Source: CAD feature listing. Evaluate the final solid. Frame: model axes, mm. A direction names the side the tool comes from. Give positions to 0.01 mm unless a question says otherwise; leave off trailing zeros. Order: outer loops, then holes, each group sorted by start corner. A loop starts at its lowest first (then second) coordinate and runs counter-clockwise, first axis right, second up.
```python
from build123d import *

# Parameters (mm, degrees)
SKETCH1_W           = 203.2
SKETCH1_H           = 152.4
BOSS_EXTRUDE1_DEPTH = 63.5
SKETCH2_W           = 196.85
SKETCH2_H           = 146.05
CUT_EXTRUDE1_DEPTH  = 60.325
SKETCH5_W           = 2.54
SKETCH5_H           = 5.08
CUT_EXTRUDE3_DEPTH  = 47.625
LPATTERN1_COUNT     = 26
LPATTERN1_PITCH     = 7.62
SKETCH6_R           = 8.75
CUT_EXTRUDE4_DEPTH  = 47.625
LPATTERN2_COUNT     = 3
LPATTERN2_PITCH     = 73.66
SKETCH7_R           = 9.525
CUT_EXTRUDE6_DEPTH  = 47.625
SKETCH8_R           = 9.525
CUT_EXTRUDE7_DEPTH  = 47.625


with BuildPart() as part:
    # Sketch1 → Boss-Extrude1 (new body)
    with BuildSketch(Plane(origin=(0, 0, 0), x_dir=(1, 0, 0), z_dir=(0, 1, 0))):
        Rectangle(SKETCH1_W, SKETCH1_H)
    extrude(amount=BOSS_EXTRUDE1_DEPTH)

    # Sketch2 → Cut-Extrude1 (cut)
    with BuildSketch(Plane(origin=(0, 63.5, 0), x_dir=(1, 0, 0), z_dir=(0, 1, 0))):
        Rectangle(SKETCH2_W, SKETCH2_H)
    extrude(amount=-CUT_EXTRUDE1_DEPTH, mode=Mode.SUBTRACT)

    # Sketch5 → Cut-Extrude3 (cut)
    with BuildSketch(Plane.XY.offset(76.2)):
        with Locations((-95.25, 20.32)):
            Rectangle(SKETCH5_W, SKETCH5_H)
    cut_extrude3 = extrude(amount=-CUT_EXTRUDE3_DEPTH, mode=Mode.SUBTRACT)

    # LPattern1: Cut-Extrude3 ×26
    with Locations(*[(i * LPATTERN1_PITCH, 0, 0) for i in range(1, LPATTERN1_COUNT)]):
        add(cut_extrude3, mode=Mode.SUBTRACT)

    # Sketch6 → Cut-Extrude4 (cut)
    with BuildSketch(Plane.XY.offset(76.2)):
        with Locations((-76.2, 44.45)):
            Circle(SKETCH6_R)
    cut_extrude4 = extrude(amount=-CUT_EXTRUDE4_DEPTH, mode=Mode.SUBTRACT)

    # LPattern2: Cut-Extrude4 ×3
    with Locations(*[(i * LPATTERN2_PITCH, 0, 0) for i in range(1, LPATTERN2_COUNT)]):
        add(cut_extrude4, mode=Mode.SUBTRACT)

    # Sketch7 → Cut-Extrude6 (cut)
    with BuildSketch(Plane(origin=(101.6, 0, 0), x_dir=(0, 0, -1), z_dir=(1, 0, 0))):
        with Locations((57.15, 19.05)):
            Circle(SKETCH7_R)
    extrude(amount=-CUT_EXTRUDE6_DEPTH, mode=Mode.SUBTRACT)

    # Sketch8 → Cut-Extrude7 (cut)
    with BuildSketch(Plane(origin=(0, 0, -76.2), x_dir=(-1, 0, 0), z_dir=(0, 0, -1))):
        with Locations((-82.55, 19.05)):
            Circle(SKETCH8_R)
    extrude(amount=-CUT_EXTRUDE7_DEPTH, mode=Mode.SUBTRACT)


solid = part.part
```
1) Reachability of faces 1 (the cylindrical face through (2.16, 51.83, 74.63)), 2 (the flat face through (101.6, 31, 1)), 3 (the flat face through (-98.425, 34, 1)), 4 (the cylindrical face through (73.75, 15.4, -74.63)), 5 (the cylindrical face through (100.035, 13.254, -49.591)) from +Z, -Z, +X, -X, +Y, -Y: full face, straight path, thin tool, end or side. Return the list, or none.
Report:
face 1: +Z
face 2: +Z, -Z, +X, +Y, -Y
face 3: +Y
face 4: -Z
face 5: +X
2) Draft query along Y for faces 6 (the cylindrical face through (-84.94, 44.83, 74.63)), 7 (the flat face through (-101.6, 31, 1)), 8 (the flat face through (-1, 0, -1)), 9 (the flat face through (-1, 3.175, -1)). Return one class per face: +Y half, -Y half, draft (parallel to the pull), parting line (faces both ways), or undercut.
Report:
face 6: undercut
face 7: draft
face 8: -Y half
face 9: +Y half
3) Section query C-C, the plane z = 3.5. Return the cut outline in (x, y) (3 decimals), and give its area (3 significant figures).
Report:
outline: (-101.6, 0) - (101.6, 0) - (101.6, 63.5) - (98.425, 63.5) - (98.425, 3.175) - (-98.425, 3.175) - (-98.425, 63.5) - (-101.6, 63.5) - close
area: 1,030 mm2
4) Section query B-B, the plane y = 55.5. Return the cut outline in (x, z) (3 decimals).
Report:
outline: (-101.6, -76.2) - (101.6, -76.2) - (101.6, 76.2) - (-101.6, 76.2) - close; hole (-98.425, -73.025) - (98.425, -73.025) - (98.425, 73.025) - (-98.425, 73.025) - close
5) Material intervals for L1, parallel to Z at x = 73, y = 13 (3 decimals); L2, parallel to X at y = 33, z = -9.5 (3 decimals); L3, parallel to Y at x = -76.2, z = 75.3, sorted ascending.
Report:
L1: z = -76.2 to -73.025, 73.025 to 76.2
L2: x = -101.6 to -98.425, 98.425 to 101.6
L3: y = 0 to 35.7, 53.2 to 63.5
6) Section query A-A, the plane z = -57.15. Return the cut outline in (x, y) (3 decimals), and give its area (3 significant figures).
Report:
outline: (-101.6, 0) - (101.6, 0) - (101.6, 9.525) - (98.425, 9.525) - (98.425, 3.175) - (-98.425, 3.175) - (-98.425, 63.5) - (-101.6, 63.5) - close; (98.425, 28.575) - (101.6, 28.575) - (101.6, 63.5) - (98.425, 63.5) - close
area: 968 mm2
7) Pin query (flat end, axial travel): pin 1 (1 mm diameter, centred on x = -9, z = 24.5, fed in from +Y) (3 decimals); pin 2 (16 mm diameter, centred on x = -2.54, y = 44.45, fed in from +Z) (3 decimals). Return the tip coordinate at first contact, or that it passes through.
Report:
pin 1: stops at y = 3.175
pin 2: stops at z = -73.025
